Work out the finished part from the listing and answer in its coordinate system (mm). A direction names the side the tool comes from. Give positions to 0.01 mm unless a question says otherwise; leave off trailing zeros. Write each loop counter-clockwise with the first axis right and the second up, starting at its lowest first coordinate (ties: lowest second). Pieces come first, ordered by that corner, then holes. Notation, with made-up numbers: (-3.75, 10) -> (32.25, 10) arc R22 cw to (32.25, 28) -> close; hole circle Ø8 at (62, -1.5). An arc over 180 degrees is marked (long way). Use a Markdown table: item, result. Add a question column.
Q1. Section A-A, the plane z = 21.5 is taken. Give the vertices of the cut face in (x, y), plus the area to 3 significant figures.
Q2. Section C-C, the plane z = -17.5 is taken. Give the vertices of the cut face in (x, y).
Q3. For a pull along Z with two mould halves and no side action, classify faces 1 (the face through (-35, 2, 23)), 2 (the face through (47, 2, 5)), 3 (the face through (40, 2, -22)) as pulls with the +Z half, pulls with the -Z half, needs draft (parallel to the pull), parting line crosses it, or undercut.
Q4. Consider line 1 (X direction, y = 2.15, z = 22); line 2 (Z direction, x = 21, y = 2.7); line 3 (X direction, y = 0.85, z = -4). Determine where each line is inside the solid, lowest interval first.
Q5. For faces 4 (the face through (-47, 2, -15)), 5 (the face through (-47, 2, -5)), 6 (the face through (-20, 2, 20)), determine the directions among +Z, -Z, +X, -X, +Y, -Y from which every point of the face is accessible in a straight line to the end or side of a thin tool.
Q6. Each of these flat-tipped pins is pushed along its axis until it touches: pin 1 Ø1.5 at (x, y) = (46.5, 2) entering from -Z; pin 2 Ø0.9 at (y, z) = (1, -19.5) entering from +X; pin 3 Ø0.9 at (x, y) = (42.5, 1) entering from -Z. Where does it stop, or does it pass through?
Q7. Section B-B, the plane x = -17.5 is taken. Give the vertices of the cut face in (y, z), plus the area to 3 significant figures.
Autodesk Inventor part; units mm, degrees
ref_plane "YZ Plane" through (0, 0, 0) normal (1, 0, 0) x (0, 1, 0)
ref_plane "XZ Plane" through (0, 0, 0) normal (0, 1, 0) x (-1, 0, 0)
ref_plane "XY Plane" through (0, 0, 0) normal (0, 0, 1) x (1, 0, 0)
sketch "Sketch1" plane through (0, 0, 0) normal (0, 1, 0) x (-1, 0, 0)
  line L0 (-48.26, 25) -> (48.26, 25)
  line L1 (48.26, 25) -> (48.26, -25)
  line L2 (48.26, -25) -> (-48.26, -25)
  line L3 (-48.26, -25) -> (-48.26, 25)
  line L4 (-48.26, 25) -> (48.26, -25) construction
  line L5 (48.26, 25) -> (-48.26, -25) construction
  point P0 (0, 0)
  dimension "d0" = 96.52
  dimension "d1" = 50
extrude "Extrusion1" add sketch "Sketch1" along normal blind 3
sketch "Sketch2" plane through (0, 3, 0) normal (0, 1, 0) x (1, 0, 0)
  line L0 (48.26, 25) -> (-48.26, 25) construction
  line L1 (-5, 25) -> (5, 25)
  line L2 (5, 25) -> (5, 22)
  line L3 (5, 22) -> (-5, 22)
  line L4 (-5, 22) -> (-5, 25)
  line L5 (0, 35) -> (0, -35) construction
  point P0 (0, 0)
  dimension "d4" = 10
  dimension "d5" = 3
extrude "Extrusion2" cut sketch "Sketch2" against normal blind 3
pattern_linear "Rectangular Pattern1" count 3 spacing 20 along (-1, 0, 0) count 2 spacing 40 along (1, 0, 0) of "Extrusion2"
sketch "Sketch3" plane through (0, 3, 0) normal (0, 1, 0) x (1, 0, 0)
  line L0 (-48.26, -25) -> (48.26, -25) construction
  line L1 (-5, -25) -> (5, -25)
  line L2 (5, -25) -> (5, -20)
  line L3 (5, -20) -> (-5, -20)
  line L4 (-5, -20) -> (-5, -25)
  line L5 (0, 35) -> (0, -35) construction
  point P0 (0, 0)
  dimension "d14" = 10
  dimension "d15" = 5
extrude "Extrusion3" cut sketch "Sketch3" against normal through all
pattern_linear "Rectangular Pattern2" count 3 spacing 20 along (-1, 0, 0) count 2 spacing 40 along (1, 0, 0) of "Extrusion3"
sketch "Sketch4" plane through (0, 3, 0) normal (0, 1, 0) x (1, 0, 0)
  line L0 (-48.26, 25) -> (-48.26, -25) construction
  line L1 (-48.26, -25) -> (-48.26, 25) construction
  line L2 (-48.26, 5) -> (-45.26, 5)
  line L3 (-45.26, 5) -> (-45.26, -5)
  line L4 (-45.26, -5) -> (-48.26, -5)
  line L5 (-48.26, -5) -> (-48.26, 5)
  line L6 (67.564, 0) -> (-67.564, 0) construction
  point P0 (0, 0)
  dimension "d24" = 3
  dimension "d25" = 10
extrude "Extrusion4" cut sketch "Sketch4" against normal through all
pattern_linear "Rectangular Pattern3" count 2 spacing 20 along (0, 0, -1) count 2 spacing 40 along (0, 0, 1) of "Extrusion4"
mirror "Mirror1" about plane through (0, 0, 0) normal (1, 0, 0) of "Extrusion4", "Rectangular Pattern3"
sketch "Sketch5" plane through (0, 3, 0) normal (0, 1, 0) x (1, 0, 0)
  line L0 (-45, 22) -> (-35, 22) construction
  line L1 (-45.26, 25) -> (-45.26, 15) construction
  line L2 (-45, 22) -> (-45.26, 22)
  line L3 (-45.26, 22) -> (-45.26, 25)
  line L4 (-45.26, 25) -> (-45, 25)
  line L5 (-45, 25) -> (-45, 22)
  line L6 (-45, -25) -> (-45, -20)
  line L7 (-45.26, -25) -> (-45, -25)
  line L8 (-45, -20) -> (-45.26, -20)
  line L9 (-45.26, -20) -> (-45.26, -25)
  line L10 (-45.26, -25) -> (-45, -25)
  line L11 (-45, -25) -> (-45, -20)
  point P0 (0, 0)
extrude "Extrusion5" cut sketch "Sketch5" against normal through all
mirror "Mirror2" about plane through (0, 0, 0) normal (1, 0, 0) of "Extrusion5"
equation "\"d0\" = Module_Width"
equation "\"d1\" = Module_Depth"
equation "\"d2\" = Module_Case_Thickness"
equation "\"d4\" = Module_Case_SlotWidth"
equation "\"d5\" = Module_Case_SlotDepth"
equation "\"d6\" = Module_Case_Thickness"
equation "\"d10\" = 2 * Module_Case_SlotWidth"
equation "\"d13\" = 4 * Module_Case_SlotWidth"
equation "\"d14\" = Module_Case_SlotWidth"
equation "\"d15\" = Module_Case_BottomSlotDepth"
equation "\"d16\" = Module_Case_Thickness"
equation "\"d20\" = 2 * Module_Case_SlotWidth"
equation "\"d23\" = 4 * Module_Case_SlotWidth"
equation "\"d24\" = Module_Case_SlotDepth"
equation "\"d25\" = Module_Case_SlotWidth"
equation "\"d26\" = Module_Case_Thickness"
equation "\"d30\" = 2 * Module_Case_SlotWidth"
equation "\"d33\" = 4 * Module_Case_SlotWidth"
equation "\"RackWidth\" = 482.6"
equation "\"U\" = 44.5"
equation "\"Module_Width\" = 96.52"
equation "\"Module_Height\" = 89"
equation "\"Module_Depth\" = 50"
equation "\"Module_Case_Thickness\" = 3"
equation "\"Module_Back_Thickness\" = 5"
equation "\"Module_Case_SlotDepth\" = 3"
equation "\"Module_Case_BottomSlotDepth\" = 5"
equation "\"Module_Case_SlotWidth\" = 10"
equation "\"Module_Connector_Width\" = 6"
equation "\"Module_Connector_Depth\" = 4"
equation "\"Module_StatusIndicatorDiameter\" = 5"
properties part number "TopBottomPlate" material "Wood (Birch)"
Result set:
| question | item | result |
|---|---|---|
| 1 | outline | (-35, 0) -> (-25, 0) -> (-25, 3) -> (-35, 3) -> close; (-15, 0) -> (-5, 0) -> (-5, 3) -> (-15, 3) -> close; (5, 0) -> (15, 0) -> (15, 3) -> (5, 3) -> close; (25, 0) -> (35, 0) -> (35, 3) -> (25, 3) -> close |
| 1 | area | 120 mm2 |
| 2 | outline | (-45.26, 0) -> (45.26, 0) -> (45.26, 3) -> (-45.26, 3) -> close |
| 3 | face 1 | needs draft |
| 3 | face 2 | undercut |
| 3 | face 3 | pulls with the -Z half |
| 4 | line 1 | x = -35 to -25, -15 to -5, 5 to 15, 25 to 35 |
| 4 | line 2 | z = -22 to 20 |
| 4 | line 3 | x = -45.26 to 45.26 |
| 5 | face 4 | -Z, -X, +Y, -Y |
| 5 | face 5 | -X, +Y, -Y |
| 5 | face 6 | +Z, +Y, -Y |
| 6 | pin 1 | stops at z = -15 |
| 6 | pin 2 | stops at x = 45.26 |
| 6 | pin 3 | stops at z = -22 |
| 7 | outline | (0, -22) -> (3, -22) -> (3, 20) -> (0, 20) -> close |
| 7 | area | 126 mm2 |
